Check sheet for the modelled part. Datum: model origin and axes. Units: mm. Face numbers are marked on the shaded views. A direction names the side the tool comes from. Give positions to 0.01 mm unless a question says otherwise; leave off trailing zeros. Order: outer loops, then holes, each group sorted by start corner. A loop starts at its lowest first (then second) coordinate and runs counter-clockwise, first axis right, second up.
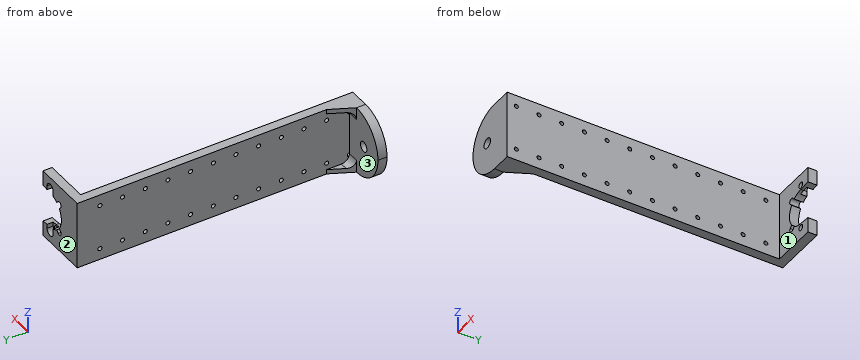
```python
from build123d import *

# Parameters (mm, degrees)
BRACKETMAINBODY_DEPTH         = 15
CUTEXTRUDE_SQUIDCUTOUTS_START = 120
SQUIDCUTOUTS_R                = 1.3
CUTEXTRUDE_SQUIDCUTOUTS_DEPTH = 244.292335528
M4_CLEARANCE_HOLE1_D          = 4.5
CUT_EXTRUDE12_REACH           = 129.189
FILLET11_R                    = 15
FILLET12_R                    = 15
F_2_56_TAPPED_HOLE1_D         = 1.778
LPATTERN3_OUTLINE_R           = 0.889
LPATTERN3_DEPTH               = 4
CUT_EXTRUDE14_START           = -2.7
CUT_EXTRUDE14_OUTLINE_R       = 1.3
CUT_EXTRUDE14_DEPTH           = 2.7
BOSS_EXTRUDE3_DEPTH           = 2
BOSS_EXTRUDE4_DEPTH           = 2
FILLET17_R                    = 3.5
FILLET18_R                    = 3.5


# Read off the part's stored shape, not the designer's step: LPattern3, Cut-Extrude14
# Some blends are built 0.0001 mm under size
with BuildPart() as part:
    # Sketch1 → BracketMainBody (new, symmetric)
    with BuildSketch(Plane.XY):
        Polygon((0, 0), (0, 120), (24, 120), (24, 116), (4, 116), (4, -4), (-20, -4), (-20, 0), align=None)
    extrude(amount=BRACKETMAINBODY_DEPTH, both=True)

    # SQUIDcutouts → CutExtrude_SQUIDcutouts (cut, through all)
    with BuildSketch(Plane(origin=(0, 0, 0), x_dir=(1, 0, 0), z_dir=(0, 1, 0)).offset(CUTEXTRUDE_SQUIDCUTOUTS_START)):
        with Locations(Location((19, -9.9, 0), (0, 0, 270))):
            Circle(SQUIDCUTOUTS_R)
        with Locations(Location((19, 9.9, 0), (0, 0, 270))):
            Circle(SQUIDCUTOUTS_R)
        with BuildLine():
            Line((12.600343686, 4.631889361), (11.616116524, 5.616116524))
            ThreePointArc((11.616116524, 5.616116524), (11.616116524, 7.383883476), (13.383883476, 7.383883476))
            Line((13.383883476, 7.383883476), (14.368110639, 6.399656314))
            ThreePointArc((14.368110639, 6.399656314), (26.9, 0), (14.368110639, -6.399656314))
            Line((14.368110639, -6.399656314), (13.383883476, -7.383883476))
            ThreePointArc((13.383883476, -7.383883476), (11.616116524, -7.383883476), (11.616116524, -5.616116524))
            Line((11.616116524, -5.616116524), (12.600343686, -4.631889361))
            ThreePointArc((12.600343686, -4.631889361), (11.1, 0), (12.600343686, 4.631889361))
        make_face()
    extrude(amount=-CUTEXTRUDE_SQUIDCUTOUTS_DEPTH, mode=Mode.SUBTRACT)

    # M4 Clearance Hole1 (through all)
    with Locations(Plane(origin=(-10, -4, 0), x_dir=(-1, 0, 0), z_dir=(0, -1, 0))):
        with Locations((0, 0)):
            Hole(M4_CLEARANCE_HOLE1_D / 2)

    # champhers<2> → Cut-Extrude12 (cut, up to next)
    with BuildSketch(Plane(origin=(0, 120, 0), x_dir=(1, 0, 0), z_dir=(0, 1, 0)), mode=Mode.PRIVATE) as cut_extrude12_sk1:
        Polygon((24, 8.337443318), (24, 6.116371473), (19, 7.9), align=None)
    cut_extrude12_tool1 = extrude(cut_extrude12_sk1.sketch, amount=-CUT_EXTRUDE12_REACH, mode=Mode.PRIVATE) & part.part
    # champhers<2> → Cut-Extrude12 (cut, up to next)
    with BuildSketch(Plane(origin=(0, 120, 0), x_dir=(1, 0, 0), z_dir=(0, 1, 0)), mode=Mode.PRIVATE) as cut_extrude12_sk2:
        Polygon((24, -6.116371473), (19, -7.9), (24, -8.337443318), align=None)
    cut_extrude12_tool2 = extrude(cut_extrude12_sk2.sketch, amount=-CUT_EXTRUDE12_REACH, mode=Mode.PRIVATE) & part.part
    add(cut_extrude12_tool1.solids().sort_by_distance((22.333333, 120, -7.451272))[0], mode=Mode.SUBTRACT)
    add(cut_extrude12_tool2.solids().sort_by_distance((22.333333, 120, 7.451272))[0], mode=Mode.SUBTRACT)

    # Fillet11
    fillet11_edges = [part.edges().sort_by_distance(p)[0] for p in [
        (-20, -2, -15),
    ]]
    fillet(fillet11_edges, radius=FILLET11_R)

    # Fillet12
    fillet12_edges = [part.edges().sort_by_distance(p)[0] for p in [
        (-20, -2, 15),
    ]]
    fillet(fillet12_edges, radius=FILLET12_R - 0.0001)  # a hair under: the kernel refuses the full size

    # #2-56 Tapped Hole1 (through all)
    with Locations(Plane(origin=(0, 110, -10), x_dir=(0, 0, -1), z_dir=(-1, 0, 0))):
        with Locations((0, 0)):
            Hole(F_2_56_TAPPED_HOLE1_D / 2)

    # LPattern3 outline → LPattern3 (cut)
    with BuildSketch(Plane.YZ):
        with Locations((110, 10)):
            Circle(LPATTERN3_OUTLINE_R)
        with Locations((100, -10)):
            Circle(LPATTERN3_OUTLINE_R)
        with Locations((100, 10)):
            Circle(LPATTERN3_OUTLINE_R)
        with Locations((90, -10)):
            Circle(LPATTERN3_OUTLINE_R)
        with Locations((90, 10)):
            Circle(LPATTERN3_OUTLINE_R)
        with Locations((80, -10)):
            Circle(LPATTERN3_OUTLINE_R)
        with Locations((80, 10)):
            Circle(LPATTERN3_OUTLINE_R)
        with Locations((70, -10)):
            Circle(LPATTERN3_OUTLINE_R)
        with Locations((70, 10)):
            Circle(LPATTERN3_OUTLINE_R)
        with Locations((60, -10)):
            Circle(LPATTERN3_OUTLINE_R)
        with Locations((60, 10)):
            Circle(LPATTERN3_OUTLINE_R)
        with Locations((50, -10)):
            Circle(LPATTERN3_OUTLINE_R)
        with Locations((50, 10)):
            Circle(LPATTERN3_OUTLINE_R)
        with Locations((40, -10)):
            Circle(LPATTERN3_OUTLINE_R)
        with Locations((40, 10)):
            Circle(LPATTERN3_OUTLINE_R)
        with Locations((30, -10)):
            Circle(LPATTERN3_OUTLINE_R)
        with Locations((30, 10)):
            Circle(LPATTERN3_OUTLINE_R)
        with Locations((20, -10)):
            Circle(LPATTERN3_OUTLINE_R)
        with Locations((20, 10)):
            Circle(LPATTERN3_OUTLINE_R)
        with Locations((10, -10)):
            Circle(LPATTERN3_OUTLINE_R)
        with Locations((10, 10)):
            Circle(LPATTERN3_OUTLINE_R)
        with Locations((0, -10)):
            Circle(LPATTERN3_OUTLINE_R)
        with Locations((0, 10)):
            Circle(LPATTERN3_OUTLINE_R)
    extrude(amount=LPATTERN3_DEPTH, mode=Mode.SUBTRACT)

    # Cut-Extrude14 outline → Cut-Extrude14 (cut)
    # profile 1 of 2: a face of its own
    with BuildSketch(Plane(origin=(0, 120, 0), x_dir=(1, 0, 0), z_dir=(0, 1, 0)).offset(CUT_EXTRUDE14_START)):
        with BuildLine():
            Line((21.124094102, -9.9), (21.124094102, -8.085834154))
            Line((21.124094102, -8.085834154), (19, -7.9))
            ThreePointArc((19, -7.9), (17.928038551, -7.82693418), (16.875905898, -7.609088267))
            Line((16.875905898, -7.609088267), (16.875905898, -9.9))
            ThreePointArc((16.875905898, -9.9), (19, -12.024094102), (21.124094102, -9.9))
        make_face()
        with Locations((19, -9.9)):
            Circle(CUT_EXTRUDE14_OUTLINE_R, mode=Mode.SUBTRACT)
    # profile 2 of 2: a face of its own
    with BuildSketch(Plane(origin=(0, 120, 0), x_dir=(1, 0, 0), z_dir=(0, 1, 0)).offset(CUT_EXTRUDE14_START)):
        with BuildLine():
            Line((21.124094102, 8.085834154), (21.124094102, 9.9))
            ThreePointArc((21.124094102, 9.9), (19, 12.024094102), (16.875905898, 9.9))
            Line((16.875905898, 9.9), (16.875905898, 7.609088267))
            ThreePointArc((16.875905898, 7.609088267), (17.928038551, 7.82693418), (19, 7.9))
            Line((19, 7.9), (21.124094102, 8.085834154))
        make_face()
        with Locations((19, 9.9)):
            Circle(CUT_EXTRUDE14_OUTLINE_R, mode=Mode.SUBTRACT)
    extrude(amount=CUT_EXTRUDE14_DEPTH, mode=Mode.SUBTRACT)

    # Sketch30 → Boss-Extrude3 (add)
    with BuildSketch(Plane.XY.offset(15)):
        Polygon((-5, 0), (0, 0), (0, 10), align=None)
    extrude(amount=-BOSS_EXTRUDE3_DEPTH)

    # Sketch31 → Boss-Extrude4 (add)
    with BuildSketch(Plane(origin=(0, 0, -15), x_dir=(-1, 0, 0), z_dir=(0, 0, -1))):
        Polygon((0, 10), (0, 0), (5, 0), align=None)
    extrude(amount=-BOSS_EXTRUDE4_DEPTH)

    # Fillet17
    # the kernel refuses this fillet: 3.5 mm, written as the material it adds along each edge
    with BuildSketch(Plane(origin=(0, 0, -13), x_dir=(0, 0, 1), z_dir=(-1, 0, 0))) as fillet17_piece_1_section:
        with BuildLine():
            CenterArc((FILLET17_R, FILLET17_R), FILLET17_R, 180, 90)
            Line((0, FILLET17_R), (0, 0))
            Line((0, 0), (FILLET17_R, 0))
        make_face()
    fillet17_piece_1 = extrude(amount=13.75, mode=Mode.PRIVATE)
    fillet17_piece_1 = split(fillet17_piece_1, bisect_by=Plane(origin=(-4.463461732, 1.073076536, -10.533039881), z_dir=(0.894427190999916, -0.44721359549995787, 0)), keep=Keep.TOP, mode=Mode.PRIVATE)
    add(fillet17_piece_1)

    # Fillet18
    # the kernel refuses this fillet: 3.5 mm, written as the material it adds along each edge
    with BuildSketch(Plane(origin=(-13.75, 0, 13), x_dir=(0, 1, 0), z_dir=(1, 0, 0))) as fillet18_piece_1_section:
        with BuildLine():
            CenterArc((FILLET18_R, -FILLET18_R), FILLET18_R, 90, 90)
            Line((0, -FILLET18_R), (0, 0))
            Line((0, 0), (FILLET18_R, 0))
        make_face()
    fillet18_piece_1 = extrude(amount=13.75, mode=Mode.PRIVATE)
    fillet18_piece_1 = split(fillet18_piece_1, bisect_by=Plane(origin=(-4.153126037, 1.693747927, 12.281398302), z_dir=(0.894427190999916, -0.447213595499958, 0)), keep=Keep.TOP, mode=Mode.PRIVATE)
    add(fillet18_piece_1)


solid = part.part
```
(1) Set-up check for the marked faces 1, 2 and 3: record each of +Z, -Z, +X, -X, +Y, -Y from which the full face is reachable in a straight line by a thin tool's end or side.
Response values:
face 1: +Z, -Z, +X, -Y
face 2: +Z, -Z, +X, -X, +Y
face 3: -X, +Y
(2) Gauge pin test, flat ends, axial feed: pin 1 Ø6 at (x, z) = (14, 4.5) entering from -Y; pin 2 Ø2.5 at (y, z) = (50, 10) entering from -X; pin 3 Ø3 at (y, z) = (50, -10) entering from +X; pin 4 Ø1.4 at (y, z) = (80, -10) entering from +X. Record the tip position at first contact, or that the pin passes through.
Response values:
pin 1: stops at y = 116
pin 2: stops at x = 0
pin 3: stops at x = 4
pin 4: passes through
(3) Material ranges on L1, parallel to Z at x = 1.3, y = 30; L2, parallel to Z at x = 19, y = 116.9; L3, parallel to X at y = 40, z = -0.5, recorded low to high.
Response values:
L1: z = -15 to -10.89, -9.11 to 9.11, 10.89 to 15
L2: z = -15 to -11.2, -8.6 to -7.9, 7.9 to 8.6, 11.2 to 15
L3: x = 0 to 4
(4) Cross-section at D-D on x = 7. Enter the section's corners in (y, z).
Response values:
outline: (116, -15) - (120, -15) - (120, 15) - (116, 15) - close
(5) Cross-section at A-A on x = -1.5. Enter the section's corners in (y, z).
Response values:
outline: (-4, -15) - (7, -15) - (7, -13) - (3.5, -13) arc R3.5 cw to (0, -9.5) - (0, 9.5) arc R3.5 cw to (3.5, 13) - (7, 13) - (7, 15) - (-4, 15) - close
(6) Cross-section at B-B on y = 5.5. Enter the section's corners in (x, z), then the cut area to 3 significant figures.
Response values:
outline: (-2.25, -15) - (4, -15) - (4, 15) - (-2.25, 15) - (-2.25, 13) - (0, 13) - (0, -13) - (-2.25, -13) - close
area: 129 mm2
(7) Cross-section at C-C on y = 24.5. Enter the section's corners in (x, z), then the cut area to 3 significant figures.
Response values:
outline: (0, -15) - (4, -15) - (4, 15) - (0, 15) - close
area: 120 mm2
